```python
from build123d import *

# Parameters (mm, degrees)
SKETCH1_R                 = 1.75
SKETCH1_R_2               = 1.525
SKETCH1_R_3               = 1.55
MAIN_FLANGE_DEPTH         = 5
SKETCH2_W                 = 15
SKETCH2_H                 = 45
SKETCH2_R                 = 1.525
SIDE_FLANGE_DEPTH         = 5
SKETCH11_R                = 1.3
BOSS_EXTRUDE3_DEPTH       = 3
BOSS_EXTRUDE4_DEPTH       = 7
SKETCH16_R                = 1.3
TOP_SUPPORT_DEPTH         = 3
SKETCH18_W                = 15
SKETCH18_H                = 8
SKETCH18_R                = 1.525
BOSS_EXTRUDE5_DEPTH       = 15
SKETCH19_W                = 15
SKETCH19_H                = 8
SKETCH19_R                = 1.525
BOSS_EXTRUDE6_DEPTH       = 15
FILLET1_R                 = 5
M3X0_5_TAPPED_HOLE1_D     = 2.6
M3X0_5_TAPPED_HOLE1_DEPTH = 7.5
M3X0_5_TAPPED_HOLE1_TIP   = 0.781118805
M3X0_5_TAPPED_HOLE2_D     = 2.6
M3X0_5_TAPPED_HOLE2_DEPTH = 7.5
M3X0_5_TAPPED_HOLE2_TIP   = 0.781118805
SKETCH24_R                = 2.5
CUT_EXTRUDE1_DEPTH        = 0.75
SKETCH25_R                = 2.5
CUT_EXTRUDE2_DEPTH        = 0.75
SKETCH26_W                = 10
SKETCH26_H                = 2.85
BOSS_EXTRUDE7_DEPTH       = 10
MOTOR_MOUNT_DEPTH         = 9
SKETCH33_W                = 15
SKETCH33_H                = 30
CUT_EXTRUDE6_DEPTH        = 2.1
SKETCH34_R                = 0.875
CUT_EXTRUDE7_DEPTH        = 7
BOSS_EXTRUDE9_DEPTH       = 9
SKETCH36_W                = 15
SKETCH36_H                = 29.05
CUT_EXTRUDE8_DEPTH        = 2.1
SKETCH37_R                = 0.875
CUT_EXTRUDE9_DEPTH        = 7
SKETCH39_W                = 45
SKETCH39_H                = 10
CUT_EXTRUDE11_DEPTH       = 52
SKETCH40_R                = 1.375
MOUNT_HOLES_DEPTH         = 4.0000001
SKETCH41_R                = 3
BEARING_HOLDER_DEPTH      = 2
SKETCH42_R                = 3
CUT_EXTRUDE14_DEPTH       = 2


with BuildPart() as part:
    # Sketch1 → main flange (new body)
    with BuildSketch(Plane.XY):
        Polygon((-22.5, 7), (0, 7), (22.5, 7), (22.5, 45), (42.5, 45), (42.5, 0), (-42.5, 0), (-42.5, 45), (-22.5, 45), align=None)
        with Locations((35.5, 8)):
            Circle(SKETCH1_R, mode=Mode.SUBTRACT)
        with Locations((-35.5, 8)):
            Circle(SKETCH1_R_2, mode=Mode.SUBTRACT)
        with Locations((32.5, 35)):
            Circle(SKETCH1_R_3, mode=Mode.SUBTRACT)
        with Locations((-32.5, 35)):
            Circle(SKETCH1_R_3, mode=Mode.SUBTRACT)
    extrude(amount=MAIN_FLANGE_DEPTH)

    # Sketch2 → side flange (add)
    with BuildSketch(Plane(origin=(22.5, 0, 0), x_dir=(0, 0, -1), z_dir=(1, 0, 0))):
        with Locations((-12.5, 22.5)):
            Rectangle(SKETCH2_W, SKETCH2_H)
        with Locations((-13, 23)):
            Circle(SKETCH2_R, mode=Mode.SUBTRACT)
        with Locations((-10, 35)):
            Circle(SKETCH2_R, mode=Mode.SUBTRACT)
    side_flange = extrude(amount=SIDE_FLANGE_DEPTH)

    # Mirror1: side flange across plane
    add(side_flange.mirror(Plane(origin=(0, 0, 0), x_dir=(0, 0, 1), z_dir=(1, 0, 0))))

    # Sketch11 → Boss-Extrude3 (add)
    with BuildSketch(Plane.XZ):
        with BuildLine():
            Line((-42.5, 0), (42.5, 0))
            Line((42.5, 0), (42.5, 10))
            ThreePointArc((42.5, 10), (39.571067812, 17.071067812), (32.5, 20))
            Line((32.5, 20), (-32.5, 20))
            ThreePointArc((-32.5, 20), (-39.571067812, 17.071067812), (-42.5, 10))
            Line((-42.5, 10), (-42.5, 0))
        make_face()
        with Locations((-32.5, 10)):
            Circle(SKETCH11_R, mode=Mode.SUBTRACT)
        with Locations((32.5, 10)):
            Circle(SKETCH11_R, mode=Mode.SUBTRACT)
    extrude(amount=BOSS_EXTRUDE3_DEPTH)

    # Sketch12 → Boss-Extrude4 (add)
    with BuildSketch(Plane(origin=(0, 0, 0), x_dir=(1, 0, 0), z_dir=(0, 1, 0))):
        with BuildLine():
            Line((-4, -3), (-4, 0))
            Line((-4, 0), (4, 0))
            Line((4, 0), (4, -3))
            ThreePointArc((4, -3), (0, -7), (-4, -3))
        make_face()
    extrude(amount=BOSS_EXTRUDE4_DEPTH)

    # Sketch15 → CSK for M3 Flat Head Machine Screw1 (revolve, cut)
    with BuildSketch(Plane(origin=(0, -3, 3), x_dir=(0, 0, -1), z_dir=(1, 0, 0))):
        Polygon((0, 0), (0, 10), (1.8, 10), (1.8, 1.5), (3.15, 0.15), (3.15, 0), align=None)
    revolve(axis=Axis((0, -9.35, 3), (0, 1, 0)), mode=Mode.SUBTRACT)

    # Sketch16 → Top support (add)
    with BuildSketch(Plane(origin=(0, 45, 0), x_dir=(1, 0, 0), z_dir=(0, 1, 0))):
        with BuildLine():
            Line((-42.5, 0), (-22.5, 0))
            Line((-22.5, 0), (-22.5, -20))
            Line((-22.5, -20), (-32.5, -20))
            ThreePointArc((-32.5, -20), (-39.571067812, -17.071067812), (-42.5, -10))
            Line((-42.5, -10), (-42.5, 0))
        make_face()
        with Locations((-32.5, -10)):
            Circle(SKETCH16_R, mode=Mode.SUBTRACT)
        with BuildLine():
            Line((42.5, 0), (42.5, -10))
            ThreePointArc((42.5, -10), (39.571067812, -17.071067812), (32.5, -20))
            Line((32.5, -20), (22.5, -20))
            Line((22.5, -20), (22.5, 0))
            Line((22.5, 0), (42.5, 0))
        make_face()
        with Locations((32.5, -10)):
            Circle(SKETCH16_R, mode=Mode.SUBTRACT)
    extrude(amount=TOP_SUPPORT_DEPTH)

    # Sketch18 → Boss-Extrude5 (add)
    with BuildSketch(Plane(origin=(27.5, 0, 0), x_dir=(0, 0, -1), z_dir=(1, 0, 0))):
        with Locations((-12.5, 23)):
            Rectangle(SKETCH18_W, SKETCH18_H)
        with Locations((-13, 23)):
            Circle(SKETCH18_R, mode=Mode.SUBTRACT)
    extrude(amount=BOSS_EXTRUDE5_DEPTH)

    # Sketch19 → Boss-Extrude6 (add)
    with BuildSketch(Plane.XY.offset(5)):
        with Locations((-35, 8)):
            Rectangle(SKETCH19_W, SKETCH19_H)
        with Locations((-35.5, 8)):
            Circle(SKETCH19_R, mode=Mode.SUBTRACT)
    extrude(amount=BOSS_EXTRUDE6_DEPTH)

    # Fillet1
    fillet1_edges = [part.edges().sort_by_distance(p)[0] for p in [
        (42.5, 23, 20),
        (-42.5, 8, 20),
    ]]
    fillet(fillet1_edges, radius=FILLET1_R)

    # M3x0.5 Tapped Hole1
    with Locations(Plane.ZY.offset(42.5)):
        with Locations((11, 8), (4, 8)):
            Hole(M3X0_5_TAPPED_HOLE1_D / 2, depth=M3X0_5_TAPPED_HOLE1_DEPTH)
            with Locations((0, 0, -(M3X0_5_TAPPED_HOLE1_DEPTH + M3X0_5_TAPPED_HOLE1_TIP / 2))):  # 118° drill point
                Cone(0, M3X0_5_TAPPED_HOLE1_D / 2, M3X0_5_TAPPED_HOLE1_TIP, mode=Mode.SUBTRACT)

    # M3x0.5 Tapped Hole2
    with Locations(Plane.XY.offset(20)):
        with Locations((33.5, 23), (26.5, 23)):
            Hole(M3X0_5_TAPPED_HOLE2_D / 2, depth=M3X0_5_TAPPED_HOLE2_DEPTH)
            with Locations((0, 0, -(M3X0_5_TAPPED_HOLE2_DEPTH + M3X0_5_TAPPED_HOLE2_TIP / 2))):  # 118° drill point
                Cone(0, M3X0_5_TAPPED_HOLE2_D / 2, M3X0_5_TAPPED_HOLE2_TIP, mode=Mode.SUBTRACT)

    # Sketch24 → Cut-Extrude1 (cut)
    with BuildSketch(Plane.XY.offset(5)):
        with Locations((35.5, 8)):
            Circle(SKETCH24_R)
    extrude(amount=-CUT_EXTRUDE1_DEPTH, mode=Mode.SUBTRACT)

    # Sketch25 → Cut-Extrude2 (cut)
    with BuildSketch(Plane.ZY.offset(27.5)):
        with Locations((13, 23)):
            Circle(SKETCH25_R)
    extrude(amount=-CUT_EXTRUDE2_DEPTH, mode=Mode.SUBTRACT)

    # Sketch26 → Boss-Extrude7 (add)
    with BuildSketch(Plane(origin=(0, 7, 0), x_dir=(1, 0, 0), z_dir=(0, 1, 0))):
        with Locations((-10.2, -1.425)):
            Rectangle(SKETCH26_W, SKETCH26_H)
        with Locations((10.2, -1.425)):
            Rectangle(SKETCH26_W, SKETCH26_H)
    extrude(amount=BOSS_EXTRUDE7_DEPTH)

    # Sketch32 → Motor mount (add)
    with BuildSketch(Plane.XY.offset(5)):
        Polygon((40.4, 14.05), (30.45, 14.05), (30.45, 1.95), (40.4, 1.95), (40.4, 0), (27.5, 0), (27.5, 19), (40.4, 19), align=None)
    extrude(amount=MOTOR_MOUNT_DEPTH)

    # Sketch33 → Cut-Extrude6 (cut)
    with BuildSketch(Plane(origin=(42.5, 0, 0), x_dir=(0, 0, -1), z_dir=(1, 0, 0))):
        with Locations((-12.5, 12)):
            Rectangle(SKETCH33_W, SKETCH33_H)
    extrude(amount=-CUT_EXTRUDE6_DEPTH, mode=Mode.SUBTRACT)

    # Sketch34 → Cut-Extrude7 (cut)
    with BuildSketch(Plane(origin=(40.4, 0, 0), x_dir=(0, 0, -1), z_dir=(1, 0, 0))):
        with Locations((-9.5, 16.5)):
            Circle(SKETCH34_R)
        with Locations((-9.5, -0.5)):
            Circle(SKETCH34_R)
    extrude(amount=-CUT_EXTRUDE7_DEPTH, mode=Mode.SUBTRACT)

    # Sketch35 → Boss-Extrude9 (add)
    with BuildSketch(Plane.ZY.offset(27.5)):
        Polygon((20, 29.05), (7.95, 29.05), (7.95, 16.95), (20, 16.95), (20, 12), (5, 12), (5, 33.05), (20, 33.05), align=None)
    extrude(amount=BOSS_EXTRUDE9_DEPTH)

    # Sketch36 → Cut-Extrude8 (cut)
    with BuildSketch(Plane.XY.offset(20)):
        with Locations((-35, 18.525)):
            Rectangle(SKETCH36_W, SKETCH36_H)
    extrude(amount=-CUT_EXTRUDE8_DEPTH, mode=Mode.SUBTRACT)

    # Sketch37 → Cut-Extrude9 (cut)
    with BuildSketch(Plane.XY.offset(17.9)):
        with Locations((-32, 31.5)):
            Circle(SKETCH37_R)
        with Locations((-32, 14.5)):
            Circle(SKETCH37_R)
    extrude(amount=-CUT_EXTRUDE9_DEPTH, mode=Mode.SUBTRACT)

    # Sketch39 → Cut-Extrude11 (cut, through all)
    with BuildSketch(Plane.XZ.offset(3)):
        with Locations((0, 5)):
            Rectangle(SKETCH39_W, SKETCH39_H)
    extrude(amount=-CUT_EXTRUDE11_DEPTH, mode=Mode.SUBTRACT)

    # Sketch40 → Mount Holes (cut, through all)
    with BuildSketch(Plane(origin=(0, 0, 0), x_dir=(1, 0, 0), z_dir=(0, 1, 0))):
        with Locations((-17.5, -15)):
            Circle(SKETCH40_R)
        with Locations((-7.5, -15)):
            Circle(SKETCH40_R)
        with Locations((7.5, -15)):
            Circle(SKETCH40_R)
        with Locations((17.5, -15)):
            Circle(SKETCH40_R)
    extrude(amount=-MOUNT_HOLES_DEPTH, mode=Mode.SUBTRACT)

    # Sketch41 → Bearing Holder (cut)
    with BuildSketch(Plane(origin=(-22.5, 0, 0), x_dir=(0, 0, -1), z_dir=(1, 0, 0))):
        with Locations((-13, 23)):
            Circle(SKETCH41_R)
    extrude(amount=-BEARING_HOLDER_DEPTH, mode=Mode.SUBTRACT)

    # Sketch42 → Cut-Extrude14 (cut)
    with BuildSketch(Plane(origin=(0, 0, 0), x_dir=(-1, 0, 0), z_dir=(0, 0, -1))):
        with Locations((-35.5, 8)):
            Circle(SKETCH42_R)
    extrude(amount=-CUT_EXTRUDE14_DEPTH, mode=Mode.SUBTRACT)


solid = part.part
```
Input: part model. Units: mm. Frame: model coordinates. A direction names the side the tool comes from. Coordinates: 2 decimals unless noted, no trailing zeros. Loops run counter-clockwise (first coordinate to the right, second up) from the corner with the lowest first, then second, coordinate; pieces in that order, holes last. Notation, with made-up numbers: M 36,75.25 L 74,75.25 A26 cw 74,93.25 Z; hole C 25.25,75 d3. An arc over 180 degrees is marked long. Answer in a Markdown table with one row per item.
1. Material intervals for line 1 (Y direction, x = 25.45, z = 10) (3 decimals); line 2 (Y direction, x = -36.5, z = 19); line 3 (X direction, y = 17, z = 15), sorted ascending.
Response:
| item | result |
|---|---|
| line 1 | y = -3 to 33.475, 36.525 to 48 |
| line 2 | y = -3 to 0, 45 to 48 |
| line 3 | x = -27.5 to -22.5, 22.5 to 27.5 |
2. First-contact query: pin 1 (2.5 mm diameter, centred on y = 8, z = 4, fed in from -X); pin 2 (5.5 mm diameter, centred on x = 35.5, y = 8, fed in from +Z); pin 3 (1.2 mm diameter, centred on x = -32, y = 31, fed in from +Z); pin 4 (1.8 mm diameter, centred on y = 23, z = 13, fed in from -X) (3 decimals). Flat tips, straight axial feed; report the tip coordinate or a pass-through.
Response:
| item | result |
|---|---|
| pin 1 | stops at x = -34.63 |
| pin 2 | stops at z = 5 |
| pin 3 | stops at z = 17.9 |
| pin 4 | passes through |
3. Draft query along X for faces 5 (the flat face through (-32, 33.05, 11)), 6 (the flat face through (30.45, 8, 9)), 7 (the flat face through (0, 0, 15)). Return one class per face: pulls with the +X half, pulls with the -X half, needs draft (parallel to the pull), parting line crosses it, or undercut.
Response:
| item | result |
|---|---|
| face 5 | needs draft |
| face 6 | pulls with the +X half |
| face 7 | undercut |
4. Section A-A, the plane y = 31.5. Output: boundary loops of the cut face in (x, z) (3 decimals).
Response:
| item | result |
|---|---|
| outline | M -42.5,0 L -22.5,0 L -22.5,20 L -27.5,20 L -27.5,17.9 L -31.125,17.9 L -31.125,10.9 L -32.875,10.9 L -32.875,17.9 L -36.5,17.9 L -36.5,5 L -42.5,5 Z; M 22.5,0 L 42.5,0 L 42.5,5 L 27.5,5 L 27.5,20 L 22.5,20 Z |
5. Section D-D, the plane x = -3. Output: boundary loops of the cut face in (y, z), then the cut area to 3 significant figures.
Response:
| item | result |
|---|---|
| outline | M -3,10 L 0,10 L 0,20 L -3,20 Z |
| area | 30.0 mm2 |
6. Section C-C, the plane y = 44. Output: boundary loops of the cut face in (x, z), then the cut area to 3 significant figures.
Response:
| item | result |
|---|---|
| outline | M -42.5,0 L -22.5,0 L -22.5,20 L -27.5,20 L -27.5,5 L -42.5,5 Z; M 22.5,0 L 42.5,0 L 42.5,5 L 27.5,5 L 27.5,20 L 22.5,20 Z |
| area | 350 mm2 |
7. Reachability of faces 1 (the cylindrical face through (37.81, 7.04, 4.63)), 2 (the cylindrical face through (-33.8, 46.48, 9.94)), 3 (the flat face through (-35, 45, 12)), 4 (the flat face through (33.4, 17, 10)) from +Z, -Z, +X, -X, +Y, -Y: full face, straight path, thin tool, end or side. Return the list, or none.
Response:
| item | result |
|---|---|
| face 1 | +Z |
| face 2 | +Y |
| face 3 | +Z, -X |
| face 4 | +X |
8. Section B-B, the plane x = 7.5. Output: boundary loops of the cut face in (y, z) (3 decimals).
Response:
| item | result |
|---|---|
| outline | M -3,10 L 0,10 L 0,13.625 L -3,13.625 Z; M -3,16.375 L 0,16.375 L 0,20 L -3,20 Z |
